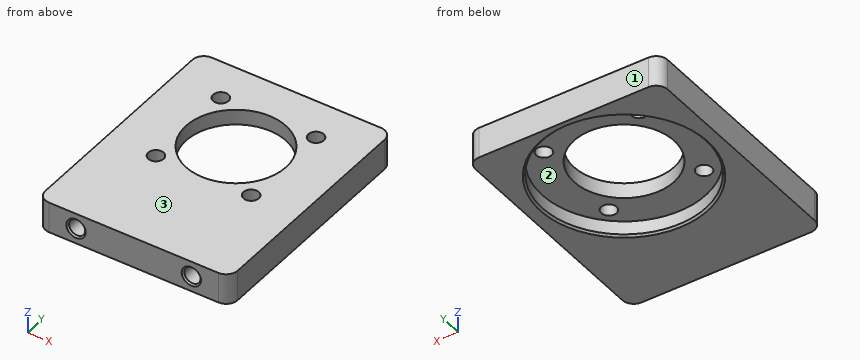
```python
from build123d import *

# Parameters (mm, degrees)
SKETCH_1_W                   = 50
SKETCH_1_H                   = 62
EXTRUDE_1_DEPTH              = 8
SKETCH_2_R                   = 13
SKETCH_2_R_2                 = 2
CUT_EXTRUDE_1_DEPTH          = 41.620192023
HOLE_WIZARD_M5_1_D           = 4.2
HOLE_WIZARD_M5_1_DEPTH       = 15
HOLE_WIZARD_M5_1_CSINK_D     = 5.05
HOLE_WIZARD_M5_1_CSINK_ANGLE = 90
HOLE_WIZARD_M5_1_TIP         = 1.2618073
FILLET_1_R                   = 3
SKETCH_6_R                   = 21.25
CUT_EXTRUDE_2_DEPTH          = 4
CHAMFER_1_SIZE               = 0.5


with BuildPart() as part:
    # 草图1 → 凸台-拉伸1 (new body)
    with BuildSketch(Plane.XY):
        Rectangle(SKETCH_1_W, SKETCH_1_H)
    extrude(amount=EXTRUDE_1_DEPTH)

    # 草图2 → 切除-拉伸1 (cut, through all)
    with BuildSketch(Plane.XY.offset(8)):
        with Locations((0, 8)):
            Circle(SKETCH_2_R)
        with Locations((12.374368671, 20.374368671)):
            Circle(SKETCH_2_R_2)
        with Locations((12.374368671, -4.374368671)):
            Circle(SKETCH_2_R_2)
        with Locations((-12.374368671, -4.374368671)):
            Circle(SKETCH_2_R_2)
        with Locations((-12.374368671, 20.374368671)):
            Circle(SKETCH_2_R_2)
    extrude(amount=-CUT_EXTRUDE_1_DEPTH, mode=Mode.SUBTRACT)

    # M5 螺纹孔1
    with Locations(Plane(origin=(-15, -31, 4), x_dir=(0, 0, -1), z_dir=(0, -1, 0))):
        with Locations((0, 0), (0, 30)):
            CounterSinkHole(HOLE_WIZARD_M5_1_D / 2, HOLE_WIZARD_M5_1_CSINK_D / 2, depth=HOLE_WIZARD_M5_1_DEPTH, counter_sink_angle=HOLE_WIZARD_M5_1_CSINK_ANGLE)
            with Locations((0, 0, -(HOLE_WIZARD_M5_1_DEPTH + HOLE_WIZARD_M5_1_TIP / 2))):  # 118° drill point
                Cone(0, HOLE_WIZARD_M5_1_D / 2, HOLE_WIZARD_M5_1_TIP, mode=Mode.SUBTRACT)

    # 圆角1
    fillet_1_edges = [part.edges().sort_by_distance(p)[0] for p in [
        (25, -31, 4),
        (-25, -31, 4),
        (-25, 31, 4),
        (25, 31, 4),
    ]]
    fillet(fillet_1_edges, radius=FILLET_1_R)

    # 草图6 → 切除-拉伸2 (cut)
    with BuildSketch(Plane(origin=(0, 0, 0), x_dir=(-1, 0, 0), z_dir=(0, 0, -1))):
        with Locations((0, 8)):
            Circle(SKETCH_6_R)
    extrude(amount=-CUT_EXTRUDE_2_DEPTH, mode=Mode.SUBTRACT)

    # 倒角1
    chamfer_1_edges = [part.edges().sort_by_distance(p)[0] for p in [
        (21.25, 8, 0),
    ]]
    chamfer(chamfer_1_edges, length=CHAMFER_1_SIZE)


solid = part.part
```
Verification items for the finished model (mm, model axes). Face numbers are marked on the shaded views. Round coordinates to 2 decimals unless told otherwise and drop trailing zeros. Order: outer loops, then holes, each group sorted by start corner. A loop starts at its lowest first (then second) coordinate and runs counter-clockwise, first axis right, second up. Notation, with made-up numbers: (4, 18) -> (23, 18) arc R28 ccw to (23, 57) -> close; hole circle Ø10 at (83, 47.25). An arc over 180 degrees is marked (long way). Put each result on its own line as item: value. Start each with the question number.
(1) Draft check along Y on the marked faces 1, 2 and 3. Enter one of: +Y half, -Y half, draft (parallel to the pull), parting line (faces both ways), or undercut.
(2) Section check A-A (x = 0). Enter the section's corners in (y, z), then the cut area to 3 significant figures.
(3) Section check D-D (x = 11.5). State how many separate pieces and enclosed holes the cut face has, then the cut area to 3 significant figures.
(4) Depth check by flat-ended pin: pin 1 Ø2.5 at (x, y) = (-12.37, -4.37) entering from -Z; pin 2 Ø2 at (x, y) = (-7, -11.5) entering from -Z. Enter the tip coordinate at first touch or a pass-through.
(5) Section check B-B (y = 8). Enter the section's corners in (x, z), then the cut area to 3 significant figures.
(6) Material ranges on line 1 along X through (y, z) = (-18.75, 4); line 2 along Z through (x, y) = (15, -22); line 3 along Y through (x, z) = (0.5, 5.25), recorded low to high.
(7) Section check C-C (y = -21). Enter the section's corners in (x, z), then the cut area to 3 significant figures.
Completed:
1. face 1: +Y half
1. face 2: undercut
1. face 3: draft
2. outline: (-31, 0) -> (-13.75, 0) -> (-13.25, 0.5) -> (-13.25, 4) -> (-5, 4) -> (-5, 8) -> (-31, 8) -> close; (21, 4) -> (29.25, 4) -> (29.25, 0.5) -> (29.75, 0) -> (31, 0) -> (31, 8) -> (21, 8) -> close
2. area: 222 mm2
3. separate pieces: 4
3. enclosed holes: 0
3. area: 275 mm2
4. pin 1: passes through
4. pin 2: stops at z = 0.03
5. outline: (-25, 0) -> (-21.75, 0) -> (-21.25, 0.5) -> (-21.25, 4) -> (-13, 4) -> (-13, 8) -> (-25, 8) -> close; (13, 4) -> (21.25, 4) -> (21.25, 0.5) -> (21.75, 0) -> (25, 0) -> (25, 8) -> (13, 8) -> close
5. area: 126 mm2
6. line 1: x = -25 to -17.1, -12.9 to 12.9, 17.1 to 25
6. line 2: z = 0 to 1.9, 6.1 to 8
6. line 3: y = -31 to -4.99, 20.99 to 31
7. outline: (-25, 0) -> (25, 0) -> (25, 8) -> (-25, 8) -> close; hole circle Ø4.2 at (-15, 4); hole circle Ø4.2 at (15, 4)
7. area: 372 mm2
